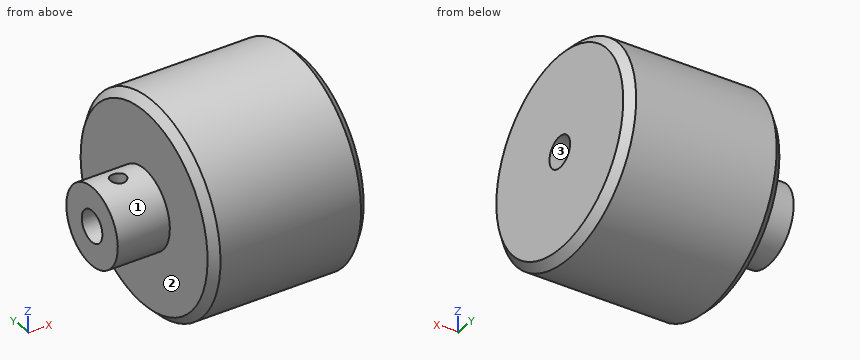
```python
from build123d import *

# Parameters (mm, degrees)
F2_SIZE2 = 15
F2_SIZE  = 15
F5_D     = 30
F5_DEPTH = 75


with BuildPart() as f1:
    # F0 (on Front) → F1 (revolve)
    with BuildSketch(Plane.XZ):
        Polygon((-200, 30), (200, 30), (200, 200), (-100, 200), (-100, 75), (-200, 75), align=None)
    revolve(axis=Axis((14.209643, 0, 0), (1, 0, 0)))

    # F2
    f2_edges = [f1.edges().sort_by_distance(p)[0] for p in [
        (-100, 0, -200),
        (200, 0, -200),
    ]]
    chamfer(f2_edges, length=F2_SIZE, length2=F2_SIZE2)

    # F5
    with Locations(Plane.XY.offset(75)):
        with Locations((-150, 0)):
            Hole(F5_D / 2, depth=F5_DEPTH)


solid = f1.part
```
Can you work these out from the model? Positions are in its coordinate system, mm. Face numbers are marked on the shaded views. Round coordinates to 2 decimals unless told otherwise and drop trailing zeros. Loops run counter-clockwise (first coordinate to the right, second up) from the corner with the lowest first, then second, coordinate; pieces in that order, holes last. Notation, with made-up numbers: M -20,-16 L 39,-16 A26 ccw 39,20 Z; hole C -13.5,75.25 d6. An arc over 180 degrees is marked long. Write item = value, one per line. Start each with the question number.
(1) Suppose I cut it at D-D on x = -36. Write out the boundary of the cut face in (y, z), plus the area to 3 significant figures.
(2) Suppose I cut it at B-B on z = 0. Write out the boundary of the cut face in (x, y).
(3) If we mould it in two halves opening along Z, with no side actions, what happens to the marked faces 1, 2 and 3? For each: released by +Z, released by -Z, zero draft, split by the parting line, or undercut.
(4) Suppose I cut it at C-C on x = -94. Write out the boundary of the cut face in (y, z).
(5) I need wall thicknesses on line 1 along X through (y, z) = (0, 36); line 2 along Y through (x, z) = (78, 0). Which ranges of each line are inside material? Lowest first, please.
(6) I'm going to push flat-ended pins straight in: P1, Ø4, axis at x = -110.5, y = 35, coming from the -Z side; P2, Ø12, axis at x = 136, z = -131, coming from the +Y side; P3, Ø12, axis at x = -69, y = -134, coming from the +Z side (3 decimals). Where does each tip first touch, or does it pass through?
(7) Suppose I cut it at A-A on y = 0. Write out the boundary of the cut face in (x, z), plus the area to 3 significant figures.
Answer block:
q1.outline = C 0,0 d400; hole C 0,0 d60
q1.area = 123,000 mm²
q2.outline = M -200,-75 L -100,-75 L -100,-185 L -85,-200 L 185,-200 L 200,-185 L 200,-30 L -200,-30 Z; M -200,30 L 200,30 L 200,185 L 185,200 L -85,200 L -100,185 L -100,75 L -200,75 Z
q3.face_1 = split by the parting line
q3.face_2 = zero draft
q3.face_3 = undercut
q4.outline = C 0,0 d382; hole C 0,0 d60
q5.line_1 = -200 to -165, -135 to 200
q5.line_2 = -200 to -30, 30 to 200
q6.P1 = -67.35
q6.P2 = 156.12
q6.P3 = 153.675
q7.outline = M -200,-75 L -100,-75 L -100,-185 L -85,-200 L 185,-200 L 200,-185 L 200,-30 L -200,-30 Z; M -200,30 L -165,30 L -165,75 L -200,75 Z; M -135,30 L 200,30 L 200,185 L 185,200 L -85,200 L -100,185 L -100,75 L -135,75 Z
q7.area = 109,000 mm²
